from build123d import *

# Parameters (mm, degrees)
F1_E2_W  = 21.512664049
F1_E2_H  = 115.1049882174
F3_DEPTH = 25.4
F4_T     = -1.524


with BuildPart() as f3:
    # F1_E2 (on explicit) → F3 (new body)
    with BuildSketch(Plane(origin=(0, 54.6783059835, 0), x_dir=(-0.5023234046, 0.8646798235, 0), z_dir=(0.8646798235, 0.5023234046, 0))):
        with Locations((10.7563320245, 57.5524941087)):
            Rectangle(F1_E2_W, F1_E2_H)
    extrude(amount=F3_DEPTH)

    # F4
    f4_openings = [f3.faces().sort_by_distance(p)[0] for p in [
        (5.578276, 70.358596, 0),
    ]]
    offset(amount=F4_T, openings=f4_openings)


solid = f3.part
The listing builds one solid part. Answer for the finished solid, in the listing's coordinates (mm). A direction names the side the tool comes from. Give positions to 0.01 mm unless a question says otherwise; leave off trailing zeros. Write each loop counter-clockwise with the first axis right and the second up, starting at its lowest first coordinate (ties: lowest second). Pieces come first, ordered by that corner, then holes. Notation, with made-up numbers: (12.25, 12) - (62.25, 12) arc R23 ccw to (62.25, 20) - close; hole circle Ø5 at (64, 40.5). An arc over 180 degrees is marked (long way). One line per question, with ' | ' between items. Start each with the question number.
1. For faces 1 (the face through (10.081, 62.297, 55.995)), 2 (the face through (16.635, 76.608, 58.358)), determine the directions among +Z, -Z, +X, -X, +Y, -Y from which every point of the face is accessible in a straight line to the end or side of a thin tool.
2. Section B-B, the plane y = 79 is taken. Determine the outline of the cut face in (x, z).
3. Section A-A, the plane z = 67.5 is taken. Determine the outline of the cut face in (x, y), then the cut area to 3 significant figures.
4. Determine the mould class of faces 3 (the face through (-5.3, 63.8, 58.4)), 4 (the face through (10, 62, 0)), 5 (the face through (15.307, 75.861, 57.586)) for opening direction X: +X half, -X half, draft (parallel to the pull), parting line (faces both ways), or undercut.
5. Given P1, Ø3, axis at y = 76, z = 56.5, coming from the +X side; P2, Ø8, axis at y = 82, z = 52.5, coming from the -X side; P3, Ø1.5, axis at y = 74.5, z = 22.5, coming from the -X side, each flat-ended and moving along its own axis, determine where each tip first touches the part or whether it passes through.
6. Section C-C, the plane x = 17 is taken. Determine the outline of the cut face in (y, z), then the cut area to 3 significant figures.
7. Straight lines are drawn through the part: line 1 (X direction, y = 66, z = 55); line 2 (X direction, y = 69.5, z = 87.5); line 3 (Y direction, x = -4.5, z = 103). For each, find the intervals that lie inside material, in ascending order.
Result:
1) face 1: -Z | face 2: +Z, -Z, +X, +Y
2) outline: (-0.96, 0) - (2.07, 0) - (2.07, 113.58) - (13.48, 113.58) - (13.48, 0) - (15.25, 0) - (15.25, 115.1) - (-0.96, 115.1) - close
3) outline: (-10.81, 73.28) - (0, 54.68) - (21.96, 67.44) - (11.16, 86.04) - close; hole (-8.72, 72.73) - (0.55, 56.76) - (19.88, 67.99) - (10.6, 83.96) - close | area: 134 mm2
4) face 3: -X half | face 4: draft | face 5: undercut
5) P1: stops at x = 17.86 | P2: stops at x = -2.68 | P3: stops at x = -10
6) outline: (64.55, 0) - (66.32, 0) - (66.32, 113.58) - (72.95, 113.58) - (72.95, 0) - (75.98, 0) - (75.98, 115.1) - (64.55, 115.1) - close | area: 562 mm2
7) line 1: x = -6.58 to -4.81, 16.45 to 19.49 | line 2: x = -8.61 to -6.85, 19 to 20.76 | line 3: y = 62.42 to 65.46, 75.18 to 76.94
